```python
from build123d import *

# Parameters (mm, degrees)
SKETCH1_W           = 12.7
SKETCH1_H           = 24
SKETCH1_R           = 1.5
BOSS_EXTRUDE1_DEPTH = 5.731831


with BuildPart() as part:
    # Sketch1 → Boss-Extrude1 (new body)
    with BuildSketch(Plane(origin=(0, -66.907851618, 0), x_dir=(-1, 0, 0), z_dir=(0, -1, 0))):
        with Locations((-55.934056303, -98.2538327)):
            Rectangle(SKETCH1_W, SKETCH1_H)
        with Locations(Location((-55.934056303, -90.2538327, 0), (0, 0, 90))):
            Circle(SKETCH1_R, mode=Mode.SUBTRACT)
        with Locations(Location((-55.934056303, -105.2538327, 0), (0, 0, 90))):
            Circle(SKETCH1_R, mode=Mode.SUBTRACT)
    extrude(amount=-BOSS_EXTRUDE1_DEPTH)


solid = part.part
```
Model file for the job. Use its own axes, mm. Round coordinates to 2 decimals unless told otherwise and drop trailing zeros. Write each loop counter-clockwise with the first axis right and the second up, starting at its lowest first coordinate (ties: lowest second). Pieces come first, ordered by that corner, then holes. Notation, with made-up numbers: (21.25, -27) - (53.25, -27) arc R8 ccw to (53.25, -15) - close; hole circle Ø4 at (-6.5, -19.5). An arc over 180 degrees is marked (long way). Use CSV: the item, a comma, the result in double quotes. Start each with the question number.
Item 1: Band-saw the part on C-C (y = -65.8). Write the cut outline in (x, z).
Item 2: Band-saw the part on D-D (z = 105.5). Write the cut outline in (x, y).
Item 3: Pin check, flat tip, straight feed: P1, Ø2.5, axis at x = 55.93, z = 90.25, coming from the -Y side. Stop position of the tip, or through.
Item 4: Band-saw the part on B-B (x = 55). Write the cut outline in (y, z).
Item 5: Two-plate mould, pull along X, no slides. Class faces 1 (the face through (49.584, -64, 98)), 2 (the face through (56.9, -64.1, 91.4)), 3 (the face through (56, -61.176, 98)): released by +X, released by -X, zero draft, split by the parting line, or undercut.
Item 6: Band-saw the part on A-A (z = 91). Write the cut outline in (x, y), and give its area (3 significant figures).
Item 7: Drill centre lines: L1, parallel to Z at x = 54.75, y = -64.1; L2, parallel to X at y = -63.75, z = 104; L3, parallel to Z at x = 57, y = -66.2. Where is each one in solid material? Low to high. Write a range as [from, to].
Checked values:
1,outline,"(49.58, 86.25) - (62.28, 86.25) - (62.28, 110.25) - (49.58, 110.25) - close; hole circle Ø3 at (55.93, 90.25); hole circle Ø3 at (55.93, 105.25)"
2,outline,"(49.58, -66.91) - (54.45, -66.91) - (54.45, -61.18) - (49.58, -61.18) - close; (57.41, -66.91) - (62.28, -66.91) - (62.28, -61.18) - (57.41, -61.18) - close"
3,P1,"passes through"
4,outline,"(-66.91, 86.25) - (-61.18, 86.25) - (-61.18, 89.08) - (-66.91, 89.08) - close; (-66.91, 91.43) - (-61.18, 91.43) - (-61.18, 104.08) - (-66.91, 104.08) - close; (-66.91, 106.43) - (-61.18, 106.43) - (-61.18, 110.25) - (-66.91, 110.25) - close"
5,face 1,"released by -X"
5,face 2,"undercut"
5,face 3,"zero draft"
6,outline,"(49.58, -66.91) - (54.63, -66.91) - (54.63, -61.18) - (49.58, -61.18) - close; (57.24, -66.91) - (62.28, -66.91) - (62.28, -61.18) - (57.24, -61.18) - close"
6,area,"57.9 mm²"
7,L1,"z = [86.25, 89.33], [91.17, 104.33], [106.17, 110.25]"
7,L2,"x = [49.58, 55.11], [56.76, 62.28]"
7,L3,"z = [86.25, 89.2], [91.31, 104.2], [106.31, 110.25]"
